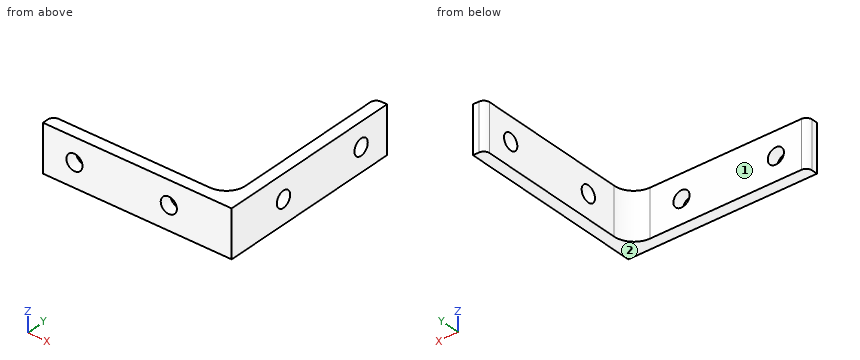
from build123d import *

# Parameters (mm, degrees)
BOSS_EXTRUDE1_DEPTH      = 9.525
F_0_257_DIAMETER_HOLE1_D = 6.5278


with BuildPart() as part:
    # Sketch2 → Boss-Extrude1 (new, symmetric)
    with BuildSketch(Plane.XY):
        with BuildLine():
            Line((-38.1, -38.1), (38.1, -38.1))
            Line((38.1, -38.1), (38.1, 38.1))
            Line((38.1, 38.1), (35.71875, 38.1))
            ThreePointArc((35.71875, 38.1), (34.034951977, 37.402548023), (33.3375, 35.71875))
            Line((33.3375, 35.71875), (33.3375, -25.4127))
            ThreePointArc((33.3375, -25.4127), (31.01637982, -31.01637982), (25.4127, -33.3375))
            Line((25.4127, -33.3375), (-35.71875, -33.3375))
            ThreePointArc((-35.71875, -33.3375), (-37.402548023, -34.034951977), (-38.1, -35.71875))
            Line((-38.1, -35.71875), (-38.1, -38.1))
        make_face()
    extrude(amount=BOSS_EXTRUDE1_DEPTH, both=True)

    # F (0.257) Diameter Hole1 (through all)
    with Locations(Plane(origin=(0, -33.3375, 0), x_dir=(1, 0, 0), z_dir=(0, 1, 0))):
        with Locations((12.7, 0), (-25.4, 0)):
            f_0_257_diameter_hole1 = Hole(F_0_257_DIAMETER_HOLE1_D / 2)

    # Mirror1: F (0.257) Diameter Hole1 across plane
    add(f_0_257_diameter_hole1.mirror(Plane(origin=(0, 0, 0), x_dir=(0, 0, 1), z_dir=(0.7071067811865474, 0.7071067811865478, 0))), mode=Mode.SUBTRACT)


solid = part.part
Read the model definition and answer for the solid it produces. Units are mm, in the model's axes. Face numbers are marked on the shaded views. A direction names the side the tool comes from. Give positions to 0.01 mm unless a question says otherwise; leave off trailing zeros. Write each loop counter-clockwise with the first axis right and the second up, starting at its lowest first coordinate (ties: lowest second). Pieces come first, ordered by that corner, then holes. Notation, with made-up numbers: (5.25, 84) - (47.25, 84) arc R32 ccw to (47.25, 116) - close; hole circle Ø3 at (22.5, 47.5). An arc over 180 degrees is marked (long way). Return JSON: item names as keys, results as strings.
Q1. A cutting plane is placed at B-B, the plane x = -25.4. Determine the outline of the cut face in (y, z) (1 decimal), and give its area (3 significant figures).
Reply:
{"outline": "(-38.1, -9.5) - (-33.3, -9.5) - (-33.3, -3.3) - (-38.1, -3.3) - close; (-38.1, 3.3) - (-33.3, 3.3) - (-33.3, 9.5) - (-38.1, 9.5) - close", "area": "59.6 mm²"}
Q2. For the marked faces 1 and 2, determine the directions among +Z, -Z, +X, -X, +Y, -Y from which every point of the face is accessible in a straight line to the end or side of a thin tool.
Reply:
{"face 1": "+Z, -Z, -X, +Y", "face 2": "-Z, +X, -X, +Y, -Y"}
Q3. A cutting plane is placed at D-D, the plane z = -5.5. Determine the outline of the cut face in (x, y).
Reply:
{"outline": "(-38.1, -38.1) - (38.1, -38.1) - (38.1, 38.1) - (35.72, 38.1) arc R2.38 ccw to (33.34, 35.72) - (33.34, -25.41) arc R7.92 cw to (25.41, -33.34) - (-35.72, -33.34) arc R2.38 ccw to (-38.1, -35.72) - close"}
Q4. Consider line 1 along Z through (x, y) = (37.15, 25.4) (3 decimals); line 2 along X through (y, z) = (1.5, 8.5); line 3 along Y through (x, z) = (21, 2.75). Determine where each line is inside the solid, lowest interval first. Write a range as [from, to].
Reply:
{"line 1": "[-9.525, -3.264], [3.264, 9.525]", "line 2": "[33.34, 38.1]", "line 3": "[-38.1, -33.34]"}
Q5. A cutting plane is placed at A-A, the plane y = -12.7. Determine the outline of the cut face in (x, z) (1 decimal), and give its area (3 significant figures).
Reply:
{"outline": "(33.3, -9.5) - (38.1, -9.5) - (38.1, -3.3) - (33.3, -3.3) - close; (33.3, 3.3) - (38.1, 3.3) - (38.1, 9.5) - (33.3, 9.5) - close", "area": "59.6 mm²"}
Q6. A cutting plane is placed at C-C, the plane z = 0. Determine the outline of the cut face in (x, y).
Reply:
{"outline": "(-38.1, -38.1) - (-28.66, -38.1) - (-28.66, -33.34) - (-35.72, -33.34) arc R2.38 ccw to (-38.1, -35.72) - close; (-22.14, -38.1) - (9.44, -38.1) - (9.44, -33.34) - (-22.14, -33.34) - close; (15.96, -38.1) - (38.1, -38.1) - (38.1, -15.96) - (33.34, -15.96) - (33.34, -25.41) arc R7.92 cw to (25.41, -33.34) - (15.96, -33.34) - close; (33.34, -9.44) - (38.1, -9.44) - (38.1, 22.14) - (33.34, 22.14) - close; (33.34, 28.66) - (38.1, 28.66) - (38.1, 38.1) - (35.72, 38.1) arc R2.38 ccw to (33.34, 35.72) - close"}
Q7. Given P1, Ø6, axis at x = 12.7, z = 0, coming from the -Y side; P2, Ø10, axis at y = 21, z = -3, coming from the -X side; P3, Ø5, axis at x = -0.5, z = -0.5, coming from the +Y side, each flat-ended and moving along its own axis, determine where each tip first touches the part or whether it passes through.
Reply:
{"P1": "through", "P2": "x = 33.34", "P3": "y = -33.34"}
